```python
from build123d import *

# Parameters (mm, degrees)
F0_W     = 57.048134
F0_H     = 46.208985
F1_DEPTH = 50.8
F2_R     = 13.918447
F3_DEPTH = 66.802
F4_R     = 7.759386
F5_DEPTH = 66.803


with BuildPart() as f1:
    # F0 (on Front) → F1 (new body)
    with BuildSketch(Plane.XZ):
        with Locations((-43.748088, 28.113147)):
            Rectangle(F0_W, F0_H)
    extrude(amount=F1_DEPTH)

    # F2 (on Front) → F3 (join)
    with BuildSketch(Plane.XZ):
        with Locations((-43.734889, 27.810963)):
            Circle(F2_R)
    extrude(amount=F3_DEPTH)

    # F4 (on Front) → F5 (cut, through all)
    with BuildSketch(Plane.XZ):
        with Locations((-43.641817, 27.810963)):
            Circle(F4_R)
    extrude(amount=F5_DEPTH, mode=Mode.SUBTRACT)


solid = f1.part
```
CAD build for the part. Positions are in the model's coordinates, mm. A direction names the side the tool comes from. Coordinates: 2 decimals unless noted, no trailing zeros. Order: outer loops, then holes, each group sorted by start corner. A loop starts at its lowest first (then second) coordinate and runs counter-clockwise, first axis right, second up. Notation, with made-up numbers: (77.25, -17) -> (88.25, -17) arc R29 ccw to (88.25, 4) -> close; hole circle Ø9 at (85.25, 9). An arc over 180 degrees is marked (long way). Use one line per item in the form item = value. Start each with the question number.
1) Pull direction Z, two halves, no side cores. Call faces 1 (the cylindrical face through (-36.24, -32.93, 30.14)), 2 (the flat face through (-15.224, -25, 28)), 3 (the flat face through (-44, -25, 5.009)): +Z half, -Z half, draft (parallel to the pull), parting line (faces both ways), or undercut.
2) Band-saw the part on C-C on y = -9. Give the cut face in (x, z), then the cut area to 3 significant figures.
3) Band-saw the part on A-A on x = -42. Give the cut face in (y, z).
4) Tool access for faces 4 (the flat face through (-44, -25, 51.218)), 5 (the cylindrical face through (-46.752, -58.689, 14.223)): list every direction of +Z, -Z, +X, -X, +Y, -Y with a clear straight run to the whole face (end or side of a thin tool).
5) Band-saw the part on D-D on x = -23.5. Give the cut face in (y, z), then the cut area to 3 significant figures.
6) Band-saw the part on B-B on z = 19. Give the cut face in (x, y), then the cut area to 3 significant figures.
7) Drill centre lines: L1, parallel to Z at x = -44.5, y = -61; L2, parallel to Z at x = -49.5, y = -17.5; L3, parallel to Y at x = -36.5, z = 42. Where is each one in solid material? Low to high. Write a range as [from, to].
8) Drop flat-ended pins along their axis: pin 1 (1 mm diameter, centred on x = -26.5, z = 30.5, fed in from +Y); pin 2 (4 mm diameter, centred on y = -55.5, z = 10.5, fed in from -X). Give the stop position or say it passes through.
Entries:
q1.face_1 = undercut
q1.face_2 = draft
q1.face_3 = -Z half
q2.outline = (-72.27, 5.01) -> (-15.22, 5.01) -> (-15.22, 51.22) -> (-72.27, 51.22) -> close; hole circle Ø15.52 at (-43.64, 27.81)
q2.area = 2,450 mm2
q3.outline = (-66.8, 14) -> (-50.8, 14) -> (-50.8, 5.01) -> (0, 5.01) -> (0, 20.23) -> (-66.8, 20.23) -> close; (-66.8, 35.39) -> (0, 35.39) -> (0, 51.22) -> (-50.8, 51.22) -> (-50.8, 41.62) -> (-66.8, 41.62) -> close
q4.face_4 = +Z, +X, -X, +Y, -Y
q4.face_5 = -Y
q5.outline = (-50.8, 5.01) -> (0, 5.01) -> (0, 51.22) -> (-50.8, 51.22) -> close
q5.area = 2,350 mm2
q6.outline = (-72.27, -50.8) -> (-54.51, -50.8) -> (-54.51, -66.8) -> (-32.96, -66.8) -> (-32.96, -50.8) -> (-15.22, -50.8) -> (-15.22, 0) -> (-72.27, 0) -> close
q6.area = 3,240 mm2
q7.L1 = [13.91, 20.1], [35.52, 41.71]
q7.L2 = [5.01, 22.72], [32.9, 51.22]
q7.L3 = [-50.8, 0]
q8.pin_1 = 0
q8.pin_2 = through
